Autodesk Inventor part; units mm, degrees
ref_plane "YZ Plane" through (0, 0, 0) normal (1, 0, 0) x (0, 1, 0)
ref_plane "XZ Plane" through (0, 0, 0) normal (0, 1, 0) x (-1, 0, 0)
ref_plane "XY Plane" through (0, 0, 0) normal (0, 0, 1) x (1, 0, 0)
sketch "Szkic1" plane through (0, 0, 0) normal (0, 1, 0) x (-1, 0, 0)
  line L0 (-15, 90) -> (15, 90)
  line L1 (15, 90) -> (15, -90)
  line L2 (15, -90) -> (-15, -90)
  line L3 (-15, -90) -> (-15, 90)
  line L4 (-15, 90) -> (15, -90) construction
  line L5 (15, 90) -> (-15, -90) construction
  point P0 (0, 0)
  dimension "d0" = 30
  dimension "d1" = 180
extrude "Wyciągnięcie proste1" add sketch "Szkic1" along normal blind 6
sketch "Szkic2" plane through (0, 6, 0) normal (0, 1, 0) x (1, 0, 0)
  line L0 (0, 0) -> (0, -75)
  line L1 (0, 0) -> (0, 75)
  dimension "d4" = 75
  dimension "d12" = 75
hole "Otwór1" at (0, 6, 75) at (0, 6, -75) direction (0, -1, 0) diameter 6.2 depth 33 tip angle 118
properties part number "łapa2"
The listing builds one solid part. Answer for the finished solid, in the listing's coordinates (mm). Round coordinates to 2 decimals unless told otherwise and drop trailing zeros. Write each loop counter-clockwise with the first axis right and the second up, starting at its lowest first coordinate (ties: lowest second). Pieces come first, ordered by that corner, then holes. Notation, with made-up numbers: M -24.5,52 L -5.5,52 A27 cw -5.5,71 Z; hole C 16,31 d9. An arc over 180 degrees is marked long. Write each question's results on one line, items separated by ' | '. Start each with the question number.
Item 1: Find section B-B on z = 75. Write down the section's boundary in (x, y), and give its area (3 significant figures).
Item 2: Straight lines are drawn through the part: probe 1 along Z at (x, y) = (0, 2.65); probe 2 along X at (y, z) = (2.25, 75); probe 3 along Z at (x, y) = (-2, 1.9). For each, find the intervals that lie inside material, in ascending order.
Item 3: The mould has two halves that part along Z. Classify faces 1 (the flat face through (0, 3, -90)), 2 (the cylindrical face through (-0.931, 2.958, 77.957)), 3 (the flat face through (15, 3, -1)), 4 (the flat face through (0, 3, 90)): +Z half, -Z half, draft (parallel to the pull), parting line (faces both ways), or undercut.
Item 4: Given pin 1 Ø3.5 at (x, z) = (0, 75) entering from +Y, flat-ended and moving along its own axis, determine where the tip first touches the part or whether it passes through.
Item 5: Find section A-A on x = 0. Write down the section's boundary in (y, z).
Answer block:
1) outline: M -15,0 L -3.1,0 L -3.1,6 L -15,6 Z; M 3.1,0 L 15,0 L 15,6 L 3.1,6 Z | area: 143 mm²
2) probe 1: z = -90 to -78.1, -71.9 to 71.9, 78.1 to 90 | probe 2: x = -15 to -3.1, 3.1 to 15 | probe 3: z = -90 to -77.37, -72.63 to 72.63, 77.37 to 90
3) face 1: -Z half | face 2: undercut | face 3: draft | face 4: +Z half
4) pin 1: passes through
5) outline: M 0,-90 L 6,-90 L 6,-78.1 L 0,-78.1 Z; M 0,-71.9 L 6,-71.9 L 6,71.9 L 0,71.9 Z; M 0,78.1 L 6,78.1 L 6,90 L 0,90 Z
